For this review, take the finished solid that the model builds, in its own axes (mm). Face numbers are marked on the shaded views. A direction names the side the tool comes from. Give positions to 0.01 mm unless a question says otherwise; leave off trailing zeros. Write each loop counter-clockwise with the first axis right and the second up, starting at its lowest first coordinate (ties: lowest second). Pieces come first, ordered by that corner, then holes.
1) For P1, Ø2, axis at x = -11, z = -4, coming from the -Y side; P2, Ø1.5, axis at x = -7, z = -9.5, coming from the -Y side; P3, Ø3, axis at x = -3.5, z = -1, coming from the -Y side, all flat-tipped, find the tip position at first contact; note any pin that passes through.
2) We need section C-C on y = -34. Give the boundary of the cut face in (x, z).
3) Machinability: for the marked faces 1 and 2, which of the approach directions +Z, -Z, +X, -X, +Y, -Y give a long, thin tool a straight path to every point of the face, cutting with its end or side? Answer none if there is none.
4) We need section A-A on x = 1. Give the boundary of the cut face in (y, z), and give its area (3 significant figures).
5) We need section B-B on z = 1. Give the boundary of the cut face in (x, y), and give its area (3 significant figures).
6) Draft analysis for pull direction X (two halves, no side actions). For the marked faces 3, 4, 5 and 6, state which applies: pulls with the +X half, pulls with the -X half, needs draft (parallel to the pull), parting line crosses it, or undercut.
7) Wall thickness on line 1 along X through (y, z) = (29, -1.25); line 2 along Y through (x, z) = (-3.5, 3.25); line 3 along Z through (x, y) = (36, 5): over which ranges is each line inside the solid? List them lowest first.
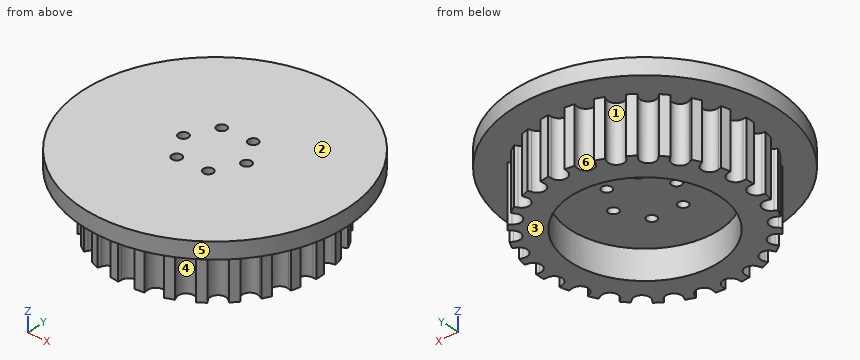
from build123d import *

# Parameters (mm, degrees)
BOSS_EXTRUDE4_DEPTH = 17
SKETCH6_R           = 40
BOSS_EXTRUDE5_DEPTH = 5
SKETCH9_R           = 22.5
CUT_EXTRUDE2_DEPTH  = 8.91448242
SKETCH10_R          = 1.5
CUT_EXTRUDE3_DEPTH  = 59.062300767


with BuildPart() as part:
    # Sketch2 → Boss-Extrude4 (new body)
    with BuildSketch(Plane.XY):
        with BuildLine():
            ThreePointArc((2.753920794, 30.877433835), (0.34063079, 28.610074808), (-2.017992552, 30.934248109))
            Line((-2.017992552, 30.934248109), (-2.126702362, 31.928321636))
            Line((-2.126702362, 31.928321636), (-4.824266539, 31.633321637))
            Line((-4.824266539, 31.633321637), (-4.715556729, 30.63924811))
            ThreePointArc((-4.715556729, 30.63924811), (-6.51610638, 27.860236315), (-9.362403491, 29.552417851))
            Line((-9.362403491, 29.552417851), (-9.705851758, 30.491589448))
            Line((-9.705851758, 30.491589448), (-12.254431503, 29.55959225))
            Line((-12.254431503, 29.55959225), (-11.910983235, 28.620420653))
            ThreePointArc((-11.910983235, 28.620420653), (-12.994151132, 25.491262155), (-16.162705571, 26.453108487))
            Line((-16.162705571, 26.453108487), (-16.72093233, 27.282796914))
            Line((-16.72093233, 27.282796914), (-18.97241345, 25.767966806))
            Line((-18.97241345, 25.767966806), (-18.414186691, 24.938278379))
            ThreePointArc((-18.414186691, 24.938278379), (-18.717023052, 21.640828495), (-22.023689951, 21.816440611))
            Line((-22.023689951, 21.816440611), (-22.764253092, 22.488427392))
            Line((-22.764253092, 22.488427392), (-24.587787689, 20.478800794))
            Line((-24.587787689, 20.478800794), (-23.847224548, 19.806814013))
            ThreePointArc((-23.847224548, 19.806814013), (-23.352129626, 16.532708544), (-26.604737525, 15.911880506))
            Line((-26.604737525, 15.911880506), (-27.48459821, 16.387112212))
            Line((-27.48459821, 16.387112212), (-28.774209082, 13.999481317))
            Line((-28.774209082, 13.999481317), (-27.894348397, 13.524249611))
            ThreePointArc((-27.894348397, 13.524249611), (-26.630095307, 10.463767667), (-29.639614458, 9.082579743))
            Line((-29.639614458, 9.082579743), (-30.607638382, 9.333437635))
            Line((-30.607638382, 9.333437635), (-31.288378032, 6.706562873))
            Line((-31.288378032, 6.706562873), (-30.320354108, 6.45570498))
            ThreePointArc((-30.320354108, 6.45570498), (-28.360416646, 3.786710647), (-30.951944734, 1.725432459))
            Line((-30.951944734, 1.725432459), (-31.951873866, 1.737337589))
            Line((-31.951873866, 1.737337589), (-31.984180179, -0.976116629))
            Line((-31.984180179, -0.976116629), (-30.984251048, -0.988021759))
            ThreePointArc((-30.984251048, -0.988021759), (-28.442533655, -3.110416231), (-30.465460488, -5.731990687))
            Line((-30.465460488, -5.731990687), (-31.43918258, -5.959730203))
            Line((-31.43918258, -5.959730203), (-30.821178033, -8.60206778))
            Line((-30.821178033, -8.60206778), (-29.847455941, -8.374328264))
            ThreePointArc((-29.847455941, -8.374328264), (-26.871673993, -9.826777024), (-28.208434416, -12.85629137))
            Line((-28.208434416, -12.85629137), (-29.09936028, -13.310440139))
            Line((-29.09936028, -13.310440139), (-27.866961049, -15.728098019))
            Line((-27.866961049, -15.728098019), (-26.976035185, -15.27394925))
            ThreePointArc((-26.976035185, -15.27394925), (-23.739130313, -15.972041255), (-24.312036669, -19.233431129))
            Line((-24.312036669, -19.233431129), (-25.068388933, -19.887595675))
            Line((-25.068388933, -19.887595675), (-23.293217582, -21.94006837))
            Line((-23.293217582, -21.94006837), (-22.536865318, -21.285903824))
            ThreePointArc((-22.536865318, -21.285903824), (-19.226954667, -21.189068505), (-19.002711722, -24.492793781))
            Line((-19.002711722, -24.492793781), (-19.58053394, -25.308956439))
            Line((-19.58053394, -25.308956439), (-17.365756976, -26.876961697))
            Line((-17.365756976, -26.876961697), (-16.787934758, -26.060799039))
            ThreePointArc((-16.787934758, -26.060799039), (-13.597378303, -25.174664112), (-12.589018241, -28.328724287))
            Line((-12.589018241, -28.328724287), (-12.954729488, -29.259452649))
            Line((-12.954729488, -29.259452649), (-10.429061697, -30.251863704))
            Line((-10.429061697, -30.251863704), (-10.063350451, -29.321135341))
            ThreePointArc((-10.063350451, -29.321135341), (-7.177571736, -27.697199747), (-5.44369678, -30.518292308))
            Line((-5.44369678, -30.518292308), (-5.576043245, -31.509495825))
            Line((-5.576043245, -31.509495825), (-2.88626726, -31.868637353))
            Line((-2.88626726, -31.868637353), (-2.753920794, -30.877433835))
            ThreePointArc((-2.753920794, -30.877433835), (-0.34063079, -28.610074808), (2.017992552, -30.934248109))
            Line((2.017992552, -30.934248109), (2.126702362, -31.928321636))
            Line((2.126702362, -31.928321636), (4.824266539, -31.633321637))
            Line((4.824266539, -31.633321637), (4.715556729, -30.63924811))
            ThreePointArc((4.715556729, -30.63924811), (6.51610638, -27.860236315), (9.362403491, -29.552417851))
            Line((9.362403491, -29.552417851), (9.705851758, -30.491589448))
            Line((9.705851758, -30.491589448), (12.254431503, -29.55959225))
            Line((12.254431503, -29.55959225), (11.910983235, -28.620420653))
            ThreePointArc((11.910983235, -28.620420653), (12.994151132, -25.491262155), (16.162705571, -26.453108487))
            Line((16.162705571, -26.453108487), (16.72093233, -27.282796914))
            Line((16.72093233, -27.282796914), (18.97241345, -25.767966806))
            Line((18.97241345, -25.767966806), (18.414186691, -24.938278379))
            ThreePointArc((18.414186691, -24.938278379), (18.717023052, -21.640828495), (22.023689951, -21.816440611))
            Line((22.023689951, -21.816440611), (22.764253092, -22.488427392))
            Line((22.764253092, -22.488427392), (24.587787689, -20.478800794))
            Line((24.587787689, -20.478800794), (23.847224548, -19.806814013))
            ThreePointArc((23.847224548, -19.806814013), (23.352129626, -16.532708544), (26.604737525, -15.911880506))
            Line((26.604737525, -15.911880506), (27.48459821, -16.387112212))
            Line((27.48459821, -16.387112212), (28.774209082, -13.999481317))
            Line((28.774209082, -13.999481317), (27.894348397, -13.524249611))
            ThreePointArc((27.894348397, -13.524249611), (26.630095307, -10.463767667), (29.639614458, -9.082579743))
            Line((29.639614458, -9.082579743), (30.607638382, -9.333437635))
            Line((30.607638382, -9.333437635), (31.288378032, -6.706562873))
            Line((31.288378032, -6.706562873), (30.320354108, -6.45570498))
            ThreePointArc((30.320354108, -6.45570498), (28.360416646, -3.786710647), (30.951944734, -1.725432459))
            Line((30.951944734, -1.725432459), (31.951873866, -1.737337589))
            Line((31.951873866, -1.737337589), (31.984180179, 0.976116629))
            Line((31.984180179, 0.976116629), (30.984251048, 0.988021759))
            ThreePointArc((30.984251048, 0.988021759), (28.442533655, 3.110416231), (30.465460488, 5.731990687))
            Line((30.465460488, 5.731990687), (31.43918258, 5.959730203))
            Line((31.43918258, 5.959730203), (30.821178033, 8.60206778))
            Line((30.821178033, 8.60206778), (29.847455941, 8.374328264))
            ThreePointArc((29.847455941, 8.374328264), (26.871673993, 9.826777024), (28.208434416, 12.85629137))
            Line((28.208434416, 12.85629137), (29.09936028, 13.310440139))
            Line((29.09936028, 13.310440139), (27.866961049, 15.728098019))
            Line((27.866961049, 15.728098019), (26.976035185, 15.27394925))
            ThreePointArc((26.976035185, 15.27394925), (23.739130313, 15.972041255), (24.312036669, 19.233431129))
            Line((24.312036669, 19.233431129), (25.068388933, 19.887595675))
            Line((25.068388933, 19.887595675), (23.293217582, 21.94006837))
            Line((23.293217582, 21.94006837), (22.536865318, 21.285903824))
            ThreePointArc((22.536865318, 21.285903824), (19.226954667, 21.189068505), (19.002711722, 24.492793781))
            Line((19.002711722, 24.492793781), (19.58053394, 25.308956439))
            Line((19.58053394, 25.308956439), (17.365756976, 26.876961697))
            Line((17.365756976, 26.876961697), (16.787934758, 26.060799039))
            ThreePointArc((16.787934758, 26.060799039), (13.597378303, 25.174664112), (12.589018241, 28.328724287))
            Line((12.589018241, 28.328724287), (12.954729488, 29.259452649))
            Line((12.954729488, 29.259452649), (10.429061697, 30.251863704))
            Line((10.429061697, 30.251863704), (10.063350451, 29.321135341))
            ThreePointArc((10.063350451, 29.321135341), (7.177571736, 27.697199747), (5.44369678, 30.518292308))
            Line((5.44369678, 30.518292308), (5.576043245, 31.509495825))
            Line((5.576043245, 31.509495825), (2.88626726, 31.868637353))
            Line((2.88626726, 31.868637353), (2.753920794, 30.877433835))
        make_face()
    extrude(amount=-BOSS_EXTRUDE4_DEPTH)

    # Sketch6 → Boss-Extrude5 (add)
    with BuildSketch(Plane.XY):
        Circle(SKETCH6_R)
    extrude(amount=BOSS_EXTRUDE5_DEPTH)

    # Sketch9 → Cut-Extrude2 (cut)
    with BuildSketch(Plane(origin=(0, 0, -17), x_dir=(-1, 0, 0), z_dir=(0, 0, -1))):
        Circle(SKETCH9_R)
    extrude(amount=-CUT_EXTRUDE2_DEPTH, mode=Mode.SUBTRACT)

    # Sketch10 → Cut-Extrude3 (cut, through all)
    with BuildSketch(Plane(origin=(0, 0, -8.08551758), x_dir=(-1, 0, 0), z_dir=(0, 0, -1))):
        with Locations((-4.744582961, 8.230366488)):
            Circle(SKETCH10_R)
        with Locations((-9.499997942, 0.006253869)):
            Circle(SKETCH10_R)
        with Locations((-4.75541498, -8.224112619)):
            Circle(SKETCH10_R)
        with Locations((4.744582961, -8.230366488)):
            Circle(SKETCH10_R)
        with Locations((9.499997942, -0.006253869)):
            Circle(SKETCH10_R)
        with Locations((4.75541498, 8.224112619)):
            Circle(SKETCH10_R)
    extrude(amount=-CUT_EXTRUDE3_DEPTH, mode=Mode.SUBTRACT)


solid = part.part
Results list:
1. P1: stops at y = -30.25
1. P2: stops at y = -28.17
1. P3: stops at y = -39.93
2. outline: (-21.07, 0) - (21.07, 0) - (21.07, 5) - (-21.07, 5) - close
3. face 1: -Z
3. face 2: +Z, +X, -X, +Y, -Y
4. outline: (-39.99, 0) - (-29.04, 0) - (-29.04, -17) - (-22.48, -17) - (-22.48, -8.09) - (22.48, -8.09) - (22.48, -17) - (28.69, -17) - (28.69, 0) - (39.99, 0) - (39.99, 5) - (-39.99, 5) - close
4. area: 981 mm2
5. outline: circle Ø80 at (0, 0); hole circle Ø3 at (-9.5, -0.01); hole circle Ø3 at (-4.76, 8.22); hole circle Ø3 at (-4.74, -8.23); hole circle Ø3 at (4.74, 8.23); hole circle Ø3 at (4.76, -8.22); hole circle Ø3 at (9.5, 0.01)
5. area: 4,980 mm2
6. face 3: needs draft
6. face 4: undercut
6. face 5: parting line crosses it
6. face 6: undercut
7. line 1: x = -12.05 to -9.13, -4.99 to -0.94, 1.68 to 5.61, 9.94 to 12.85
7. line 2: y = -39.85 to -9.07, -7.39 to 7.4, 9.05 to 39.85
7. line 3: z = 0 to 5
